Verification items for the finished model (mm, model axes). A direction names the side the tool comes from. Round coordinates to 2 decimals unless told otherwise and drop trailing zeros. Write each loop counter-clockwise with the first axis right and the second up, starting at its lowest first coordinate (ties: lowest second). Pieces come first, ordered by that corner, then holes. Notation, with made-up numbers: (18, -28.75) -> (72, -28.75) arc R25 ccw to (72, -10.75) -> close; hole circle Ø1 at (-8.5, 51.5). An arc over 180 degrees is marked (long way). Answer as a JSON object with one key per item and string values. Group by question number.
(1) Set-up check for faces 1 (the face through (0, 0, 0)), 2 (the face through (-7, 99.06, 0)): record each of +Z, -Z, +X, -X, +Y, -Y from which the full face is reachable in a straight line by a thin tool's end or side.
(2) Draft check along Z on faces 3 (the face through (-10, 104.14, -32)), 4 (the face through (-30.67, 52.16, -30.47)), 5 (the face through (0, 101, -30.48)), 6 (the face through (-30.48, 101, 0)). Enter one of: released by +Z, released by -Z, zero draft, split by the parting line, or undercut.
(3) Sectioned sample at A-A on x = 0. Record the cut outline in (y, z).
(4) Sectioned sample at C-C on y = 9.5. Record the cut outline in (x, z).
(5) Gauge pin test, flat ends, axial feed: pin 1 Ø3 at (y, z) = (63.5, 24) entering from -X; pin 2 Ø10 at (x, z) = (-22.5, 12) entering from +Y. Record the tip position at first contact, or that the pin passes through.
(6) Scan lines: L1, parallel to X at y = 103, z = 20; L2, parallel to Y at x = -25.5, z = -15.5; L3, parallel to X at y = 56, z = -22. Record each from-to range of solid material in increasing order. Write a range as from..to.
(7) Sectioned sample at B-B on z = 16.5. Record the cut outline in (x, y), and give its area (3 significant figures).
```python
from build123d import *

# Parameters (mm, degrees)
SKETCH2_W          = 68.58
SKETCH2_H          = 68.58
BASE_EXTRUDE_DEPTH = 104.14
SIDE_FILLETS_R     = 12.7
TOP_CUT_DEPTH      = 5.08
TOP_FACE_FILLET_R  = 1.27
SKETCH9_R          = 6.35
TERMINALS_DEPTH    = 15.24
TERMINALS_TAPER    = 5


with BuildPart() as part:
    # Sketch2 → Base-Extrude (new body)
    with BuildSketch(Plane(origin=(0, 0, 0), x_dir=(1, 0, 0), z_dir=(0, 1, 0))):
        Rectangle(SKETCH2_W, SKETCH2_H)
    extrude(amount=BASE_EXTRUDE_DEPTH)

    # Side Fillets
    side_fillets_edges = [part.edges().sort_by_distance(p)[0] for p in [
        (34.29, 52.07, 34.29),
        (-34.29, 52.07, 34.29),
        (-34.29, 52.07, -34.29),
        (34.29, 52.07, -34.29),
    ]]
    fillet(side_fillets_edges, radius=SIDE_FILLETS_R)

    # Sketch5 → Top Cut (cut)
    with BuildSketch(Plane(origin=(0, 104.14, 0), x_dir=(1, 0, 0), z_dir=(0, 1, 0))):
        with BuildLine():
            Line((-30.48, 21.59), (-30.48, -21.59))
            ThreePointArc((-30.48, -21.59), (-27.876179285, -27.876179285), (-21.59, -30.48))
            Line((-21.59, -30.48), (21.59, -30.48))
            ThreePointArc((21.59, -30.48), (27.876179285, -27.876179285), (30.48, -21.59))
            Line((30.48, -21.59), (30.48, 21.59))
            ThreePointArc((30.48, 21.59), (27.876179285, 27.876179285), (21.59, 30.48))
            Line((21.59, 30.48), (-21.59, 30.48))
            ThreePointArc((-21.59, 30.48), (-27.876179285, 27.876179285), (-30.48, 21.59))
        make_face()
    extrude(amount=-TOP_CUT_DEPTH, mode=Mode.SUBTRACT)

    # Top Face Fillet
    top_face_fillet_edges = [part.edges().sort_by_distance(p)[0] for p in [
        (0, 104.14, 34.29),
        (-34.29, 104.14, 0),
        (34.29, 104.14, 0),
        (0, 104.14, -34.29),
        (30.570256121, 104.14, 30.570256121),
        (30.570256121, 104.14, -30.570256121),
        (-30.570256121, 104.14, -30.570256121),
        (-30.570256121, 104.14, 30.570256121),
        (-27.876179285, 104.14, -27.876179285),
        (-30.48, 104.14, 0),
        (-27.876179285, 104.14, 27.876179285),
        (0, 104.14, 30.48),
        (27.876179285, 104.14, 27.876179285),
        (30.48, 104.14, 0),
        (27.876179285, 104.14, -27.876179285),
        (0, 104.14, -30.48),
    ]]
    fillet(top_face_fillet_edges, radius=TOP_FACE_FILLET_R)

    # Sketch9 → Terminals (add)
    with BuildSketch(Plane(origin=(0, 99.06, 0), x_dir=(1, 0, 0), z_dir=(0, 1, 0))):
        Circle(SKETCH9_R)
        with Locations((-17.960512242, 17.960512242)):
            Circle(SKETCH9_R)
    extrude(amount=TERMINALS_DEPTH, taper=TERMINALS_TAPER)


solid = part.part
```
Computed values:
{
 "1": {"face 1": "+Z, -Z, +X, -X, -Y", "face 2": "+Y"},
 "2": {"face 3": "zero draft", "face 4": "released by -Z", "face 5": "undercut", "face 6": "undercut"},
 "3": {"outline": "(0, -34.29) -> (102.87, -34.29) arc R1.27 ccw to (104.14, -33.02) -> (104.14, -31.75) arc R1.27 ccw to (102.87, -30.48) -> (99.06, -30.48) -> (99.06, -6.35) -> (114.3, -5.02) -> (114.3, 5.02) -> (99.06, 6.35) -> (99.06, 30.48) -> (102.87, 30.48) arc R1.27 ccw to (104.14, 31.75) -> (104.14, 33.02) arc R1.27 ccw to (102.87, 34.29) -> (0, 34.29) -> close"},
 "4": {"outline": "(-34.29, -21.59) arc R12.7 ccw to (-21.59, -34.29) -> (21.59, -34.29) arc R12.7 ccw to (34.29, -21.59) -> (34.29, 21.59) arc R12.7 ccw to (21.59, 34.29) -> (-21.59, 34.29) arc R12.7 ccw to (-34.29, 21.59) -> close"},
 "5": {"pin 1": "x = -34.26", "pin 2": "y = 99.06"},
 "6": {"L1": "-34.28..-30.49, 30.49..34.28", "L2": "0..99.06", "L3": "-34.28..34.28"},
 "7": {"outline": "(-34.29, 0) -> (34.29, 0) -> (34.29, 102.87) arc R1.27 ccw to (33.02, 104.14) -> (31.75, 104.14) arc R1.27 ccw to (30.48, 102.87) -> (30.48, 99.06) -> (-30.48, 99.06) -> (-30.48, 102.87) arc R1.27 ccw to (-31.75, 104.14) -> (-33.02, 104.14) arc R1.27 ccw to (-34.29, 102.87) -> close", "area": "6,830 mm2"}
}
